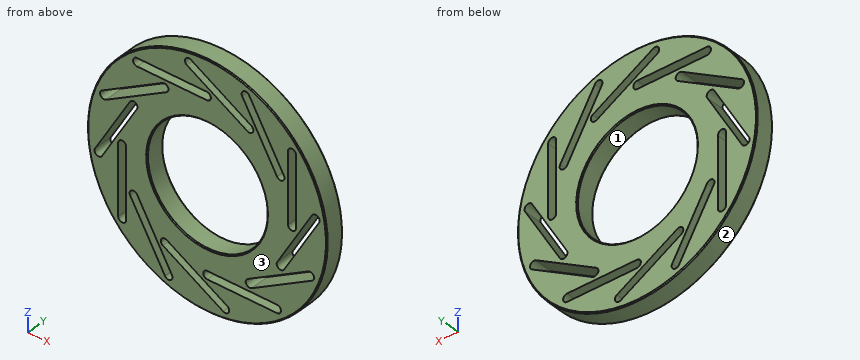
from build123d import *

# Parameters (mm, degrees)
SKETCH1_R           = 25
SKETCH1_R_2         = 12.5
BOSS_EXTRUDE1_DEPTH = 4
CHAMFER1_SIZE       = 0.2


with BuildPart() as part:
    # Sketch1 → Boss-Extrude1 (new body)
    with BuildSketch(Plane(origin=(0, 0, 0), x_dir=(1, 0, 0), z_dir=(0, 1, 0))):
        with Locations(Location((0, 0, 0), (0, 0, 270))):
            Circle(SKETCH1_R)
        with Locations(Location((0, 0, 0), (0, 0, 270))):
            Circle(SKETCH1_R_2, mode=Mode.SUBTRACT)
        with BuildLine():
            Line((16.875, -14.583333333), (16.875, -0.041666667))
            ThreePointArc((16.875, -0.041666667), (17.708333333, 0.791666667), (18.541666667, -0.041666667))
            Line((18.541666667, -0.041666667), (18.541666667, -14.583333333))
            ThreePointArc((18.541666667, -14.583333333), (17.708333333, -15.416666667), (16.875, -14.583333333))
        make_face(mode=Mode.SUBTRACT)
        with BuildLine():
            Line((16.078387695, 9.234748942), (23.349221029, -3.358703805))
            ThreePointArc((23.349221029, -3.358703805), (23.044199859, -4.497058308), (21.905845356, -4.192037139))
            Line((21.905845356, -4.192037139), (14.635012022, 8.401415608))
            ThreePointArc((14.635012022, 8.401415608), (14.940033192, 9.539770111), (16.078387695, 9.234748942))
        make_face(mode=Mode.SUBTRACT)
        with BuildLine():
            Line((7.322512022, -21.067037139), (14.593345356, -8.473584392))
            ThreePointArc((14.593345356, -8.473584392), (15.731699859, -8.168563222), (16.036721029, -9.306917725))
            Line((16.036721029, -9.306917725), (8.765887695, -21.900370472))
            ThreePointArc((8.765887695, -21.900370472), (7.627533192, -22.205391642), (7.322512022, -21.067037139))
        make_face(mode=Mode.SUBTRACT)
        with BuildLine():
            Line((-4.192037139, -21.905845356), (8.401415608, -14.635012022))
            ThreePointArc((8.401415608, -14.635012022), (9.539770111, -14.940033192), (9.234748942, -16.078387695))
            Line((9.234748942, -16.078387695), (-3.358703805, -23.349221029))
            ThreePointArc((-3.358703805, -23.349221029), (-4.497058308, -23.044199859), (-4.192037139, -21.905845356))
        make_face(mode=Mode.SUBTRACT)
        with BuildLine():
            Line((-14.583333333, -16.875), (-0.041666667, -16.875))
            ThreePointArc((-0.041666667, -16.875), (0.791666667, -17.708333333), (-0.041666667, -18.541666667))
            Line((-0.041666667, -18.541666667), (-14.583333333, -18.541666667))
            ThreePointArc((-14.583333333, -18.541666667), (-15.416666667, -17.708333333), (-14.583333333, -16.875))
        make_face(mode=Mode.SUBTRACT)
        with BuildLine():
            Line((-21.067037139, -7.322512022), (-8.473584392, -14.593345356))
            ThreePointArc((-8.473584392, -14.593345356), (-8.168563222, -15.731699859), (-9.306917725, -16.036721029))
            Line((-9.306917725, -16.036721029), (-21.900370472, -8.765887695))
            ThreePointArc((-21.900370472, -8.765887695), (-22.205391642, -7.627533192), (-21.067037139, -7.322512022))
        make_face(mode=Mode.SUBTRACT)
        with BuildLine():
            Line((-21.905845356, 4.192037139), (-14.635012022, -8.401415608))
            ThreePointArc((-14.635012022, -8.401415608), (-14.940033192, -9.539770111), (-16.078387695, -9.234748942))
            Line((-16.078387695, -9.234748942), (-23.349221029, 3.358703805))
            ThreePointArc((-23.349221029, 3.358703805), (-23.044199859, 4.497058308), (-21.905845356, 4.192037139))
        make_face(mode=Mode.SUBTRACT)
        with BuildLine():
            Line((-16.875, 14.583333333), (-16.875, 0.041666667))
            ThreePointArc((-16.875, 0.041666667), (-17.708333333, -0.791666667), (-18.541666667, 0.041666667))
            Line((-18.541666667, 0.041666667), (-18.541666667, 14.583333333))
            ThreePointArc((-18.541666667, 14.583333333), (-17.708333333, 15.416666667), (-16.875, 14.583333333))
        make_face(mode=Mode.SUBTRACT)
        with BuildLine():
            Line((-7.322512022, 21.067037139), (-14.593345356, 8.473584392))
            ThreePointArc((-14.593345356, 8.473584392), (-15.731699859, 8.168563222), (-16.036721029, 9.306917725))
            Line((-16.036721029, 9.306917725), (-8.765887695, 21.900370472))
            ThreePointArc((-8.765887695, 21.900370472), (-7.627533192, 22.205391642), (-7.322512022, 21.067037139))
        make_face(mode=Mode.SUBTRACT)
        with BuildLine():
            Line((4.192037139, 21.905845356), (-8.401415608, 14.635012022))
            ThreePointArc((-8.401415608, 14.635012022), (-9.539770111, 14.940033192), (-9.234748942, 16.078387695))
            Line((-9.234748942, 16.078387695), (3.358703805, 23.349221029))
            ThreePointArc((3.358703805, 23.349221029), (4.497058308, 23.044199859), (4.192037139, 21.905845356))
        make_face(mode=Mode.SUBTRACT)
        with BuildLine():
            Line((14.583333333, 16.875), (0.041666667, 16.875))
            ThreePointArc((0.041666667, 16.875), (-0.791666667, 17.708333333), (0.041666667, 18.541666667))
            Line((0.041666667, 18.541666667), (14.583333333, 18.541666667))
            ThreePointArc((14.583333333, 18.541666667), (15.416666667, 17.708333333), (14.583333333, 16.875))
        make_face(mode=Mode.SUBTRACT)
        with BuildLine():
            Line((21.067037139, 7.322512022), (8.473584392, 14.593345356))
            ThreePointArc((8.473584392, 14.593345356), (8.168563222, 15.731699859), (9.306917725, 16.036721029))
            Line((9.306917725, 16.036721029), (21.900370472, 8.765887695))
            ThreePointArc((21.900370472, 8.765887695), (22.205391642, 7.627533192), (21.067037139, 7.322512022))
        make_face(mode=Mode.SUBTRACT)
    extrude(amount=BOSS_EXTRUDE1_DEPTH)

    # Chamfer1
    chamfer1_edges = [part.edges().sort_by_distance(p)[0] for p in [
        (0, 0, -12.5),
        (0, 4, -12.5),
        (0, 0, -25),
        (0, 4, -25),
    ]]
    chamfer(chamfer1_edges, length=CHAMFER1_SIZE)


solid = part.part
Work out the finished part from the listing and answer in its coordinate system (mm). Face numbers are marked on the shaded views. Give positions to 0.01 mm unless a question says otherwise; leave off trailing zeros. Answer as a JSON object with one key per item and string values. Group by question number.
1. Flat-ended cylindrical pins translate along their axes: pin 1 Ø2 at (y, z) = (2, 5.5) entering from -X; pin 2 Ø2 at (y, z) = (2.5, -3.5) entering from -X; pin 3 Ø1.2 at (y, z) = (1.5, 5.5) entering from +X. Find the tip coordinate at first contact, or state that the pin passes through.
2. Consider line 1 along X through (y, z) = (3.85, 10.5) (3 decimals); line 2 along X through (y, z) = (2.15, -18); line 3 along X through (y, z) = (2.4, 0). Determine where each line is inside the solid, lowest interval first. Write a range as [from, to].
3. The mould has two halves that part along X. Classify the marked faces 1, 2 and 3: released by +X, released by -X, zero draft, split by the parting line, or undercut.
4. Section A-A on y = 2.55 is taken. Count the separate pieces of the cut face and the enclosed holes in it, plus the area to 3 significant figures.
Result sheet:
{
 "1": {"pin 1": "stops at x = -24.59", "pin 2": "stops at x = -24.87", "pin 3": "stops at x = 24.52"},
 "2": {"line 1": "x = [-22.633, -18.897], [-15.563, -6.874], [6.874, 13.423], [15.348, 16.875], [18.542, 22.633]", "line 2": "x = [-17.35, -11.02], [-9.09, -5.91], [-2.57, -0.74], [15.36, 17.35]", "line 3": "x = [-25, -21.41], [-19.49, -18.54], [-16.88, -12.5], [12.5, 16.88], [18.54, 19.49], [21.41, 25]"},
 "3": {"face 1": "undercut", "face 2": "split by the parting line", "face 3": "zero draft"},
 "4": {"separate pieces": "1", "enclosed holes": "13", "area": "1,160 mm^2"}
}
